For this review, take the finished solid that the model builds, in its own axes (mm). A direction names the side the tool comes from. Coordinates: 2 decimals unless noted, no trailing zeros. Loops run counter-clockwise (first coordinate to the right, second up) from the corner with the lowest first, then second, coordinate; pieces in that order, holes last. Notation, with made-up numbers: M -14,22.25 L -8,22.25 A30 cw -8,51.25 Z; hole C 5,-17.75 d6. An arc over 180 degrees is marked long. Put each result on its own line as item: value.
```python
from build123d import *

# Parameters (mm, degrees)
SKETCH1_R           = 50
SKETCH1_R_2         = 5
BOSS_EXTRUDE1_DEPTH = 20
SKETCH2_R           = 34.5
SKETCH2_R_2         = 33
CUT_EXTRUDE1_DEPTH  = 1.5


with BuildPart() as part:
    # Sketch1 → Boss-Extrude1 (new body)
    with BuildSketch(Plane.XY):
        Circle(SKETCH1_R)
        with Locations((0, -41)):
            Circle(SKETCH1_R_2, mode=Mode.SUBTRACT)
        with Locations((-24.099195344, -33.169696769)):
            Circle(SKETCH1_R_2, mode=Mode.SUBTRACT)
        with Locations((-38.993317168, -12.669696769)):
            Circle(SKETCH1_R_2, mode=Mode.SUBTRACT)
        with Locations((-38.993317168, 12.669696769)):
            Circle(SKETCH1_R_2, mode=Mode.SUBTRACT)
        with Locations((-24.099195344, 33.169696769)):
            Circle(SKETCH1_R_2, mode=Mode.SUBTRACT)
        with Locations((0, 41)):
            Circle(SKETCH1_R_2, mode=Mode.SUBTRACT)
        with Locations((24.099195344, 33.169696769)):
            Circle(SKETCH1_R_2, mode=Mode.SUBTRACT)
        with Locations((38.993317168, 12.669696769)):
            Circle(SKETCH1_R_2, mode=Mode.SUBTRACT)
        with Locations((38.993317168, -12.669696769)):
            Circle(SKETCH1_R_2, mode=Mode.SUBTRACT)
        with Locations((24.099195344, -33.169696769)):
            Circle(SKETCH1_R_2, mode=Mode.SUBTRACT)
    extrude(amount=BOSS_EXTRUDE1_DEPTH)

    # Sketch2 → Cut-Extrude1 (cut)
    with BuildSketch(Plane.XY.offset(20)):
        Circle(SKETCH2_R)
        Circle(SKETCH2_R_2, mode=Mode.SUBTRACT)
    extrude(amount=-CUT_EXTRUDE1_DEPTH, mode=Mode.SUBTRACT)


solid = part.part
```
(1) Add section A-A (x = 0). Write out the cut boundary in (y, z), plus the area to 3 significant figures.
Determined:
outline: M -50,0 L -46,0 L -46,20 L -50,20 Z; M -36,0 L 36,0 L 36,20 L 34.5,20 L 34.5,18.5 L 33,18.5 L 33,20 L -33,20 L -33,18.5 L -34.5,18.5 L -34.5,20 L -36,20 Z; M 46,0 L 50,0 L 50,20 L 46,20 Z
area: 1,600 mm^2
(2) Wall thickness on line 1 along Y through (x, z) = (0, 7.75); line 2 along Y through (x, z) = (0, 19.4); line 3 along Y through (x, z) = (-36.5, 19.25): over which ranges is each line inside the solid? List them lowest first. Write a range as [from, to].
Determined:
line 1: y = [-50, -46], [-36, 36], [46, 50]
line 2: y = [-50, -46], [-36, -34.5], [-33, 33], [34.5, 36], [46, 50]
line 3: y = [-34.17, -17], [-8.34, 8.34], [17, 34.17]
(3) Add section D-D (y = 24.5). Write out the cut boundary in (x, z).
Determined:
outline: M -43.59,0 L 43.59,0 L 43.59,20 L 24.29,20 L 24.29,18.5 L 22.11,18.5 L 22.11,20 L -22.11,20 L -22.11,18.5 L -24.29,18.5 L -24.29,20 L -43.59,20 Z
(4) For pin 1 (9 mm diameter, centred on x = -24.1, y = 33.17, fed in from -Z); pin 2 (1 mm diameter, centred on y = -13, z = 10.5, fed in from +X); pin 3 (5 mm diameter, centred on y = 30, z = 6.5, fed in from +X); pin 4 (3 mm diameter, centred on y = 17.5, z = 10.5, fed in from +X), all flat-tipped, find the tip position at first contact; note any pin that passes through.
Determined:
pin 1: passes through
pin 2: stops at x = 48.41
pin 3: stops at x = 41.76
pin 4: stops at x = 47.37
(5) Add section C-C (z = 13.5). State how many separate pieces and enclosed holes the cut face has, plus the area to 3 significant figures.
Determined:
separate pieces: 1
enclosed holes: 10
area: 7,070 mm^2
(6) Add section B-B (y = 41). Write out the cut boundary in (x, z).
Determined:
outline: M -28.62,0 L -5,0 L -5,20 L -28.62,20 Z; M 5,0 L 28.62,0 L 28.62,20 L 5,20 Z
(7) Tool access review of faces 1 (the cylindrical face through (23.448, 38.127, 9.86)), 2 (the cylindrical face through (32.907, 10.363, 19.26)): name each direction out of +Z, -Z, +X, -X, +Y, -Y from which nothing blocks a thin tool from reaching the whole face with its end or side.
Determined:
face 1: +Z, -Z
face 2: +Z
(8) Draft analysis for pull direction X (two halves, no side actions). For faces 3 (the flat face through (11, -33, 20)), 4 (the cylindrical face through (47.69, 15.02, 9.86)), 5 (the cylindrical face through (-43.99, 12.89, 9.86)), state which applies: +X half, -X half, draft (parallel to the pull), parting line (faces both ways), or undercut.
Determined:
face 3: draft
face 4: parting line
face 5: undercut
